Source: three-view drawing plus pictorial views. Frame: mm from the lowest corner of the part. Coordinates: 2 decimals unless noted, no trailing zeros. Write each loop counter-clockwise with the first axis right and the second up, starting at its lowest first coordinate (ties: lowest second). Pieces come first, ordered by that corner, then holes. Notation, with made-up numbers: M 0.25,19 L 23.25,19 A19 cw 23.25,54 Z; hole C 49,8 d4. An arc over 180 degrees is marked long. Use CSV: the item, a comma, the result in double quotes.
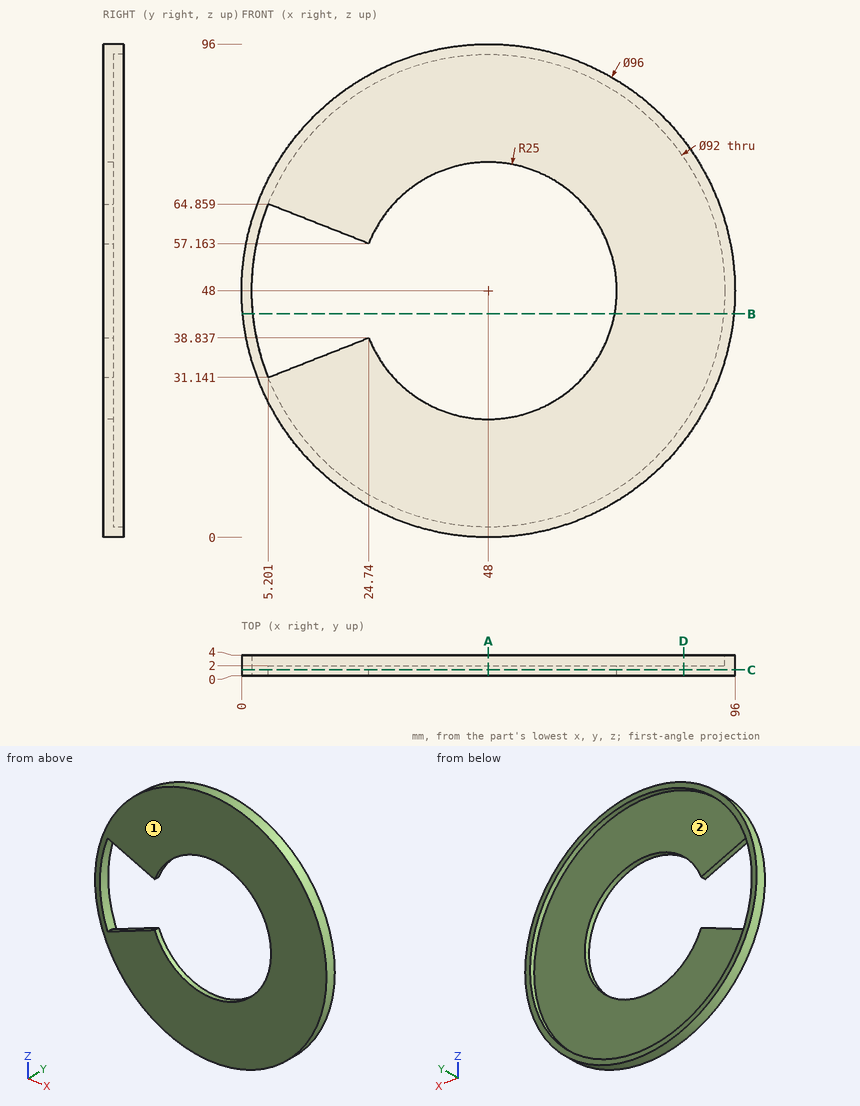
1. Section A-A (x = 48). Return loops of the section in (y, z).
Resolved:
outline,"M 0,0 L 4,0 L 4,2 L 2,2 L 2,23 L 0,23 Z; M 0,73 L 2,73 L 2,94 L 4,94 L 4,96 L 0,96 Z"
2. Section D-D (x = 86). Return loops of the section in (y, z) (1 decimal).
Resolved:
outline,"M 0,18.7 L 4,18.7 L 4,22.1 L 2,22.1 L 2,73.9 L 4,73.9 L 4,77.3 L 0,77.3 Z"
3. Section B-B (z = 43.5). Return loops of the section in (x, y).
Resolved:
outline,"M 0.21,0 L 2.22,0 L 2.22,4 L 0.21,4 Z; M 72.59,0 L 95.79,0 L 95.79,4 L 93.78,4 L 93.78,2 L 72.59,2 Z"
4. Contact query for flat-ended pins moving along their axis: pin 1 Ø5 at (x, z) = (30, 80.5) entering from +Y; pin 2 Ø1 at (y, z) = (3, 12) entering from -X. Output: stop coordinate, or through.
Resolved:
pin 1,"stops at y = 2"
pin 2,"stops at x = 15.69"
5. Section C-C (y = 1.2). Return loops of the section in (x, z).
Resolved:
outline,"C 48,48 d96; hole M 5.2,31.14 L 24.74,38.84 A25 ccw long 24.74,57.16 L 5.2,64.86 A46 ccw Z"
6. Material intervals for line 1 (X direction, y = 2.25, z = 48); line 2 (X direction, y = 1.05, z = 48), sorted ascending. Write a range as [from, to].
Resolved:
line 1,"x = [0, 2], [94, 96]"
line 2,"x = [0, 2], [73, 96]"
7. Mould query, pull axis X, two halves, no side actions, for the marked faces 1 and 2. Classes: pulls with the +X half, pulls with the -X half, needs draft (parallel to the pull), parting line crosses it, or undercut.
Resolved:
face 1,"needs draft"
face 2,"undercut"
